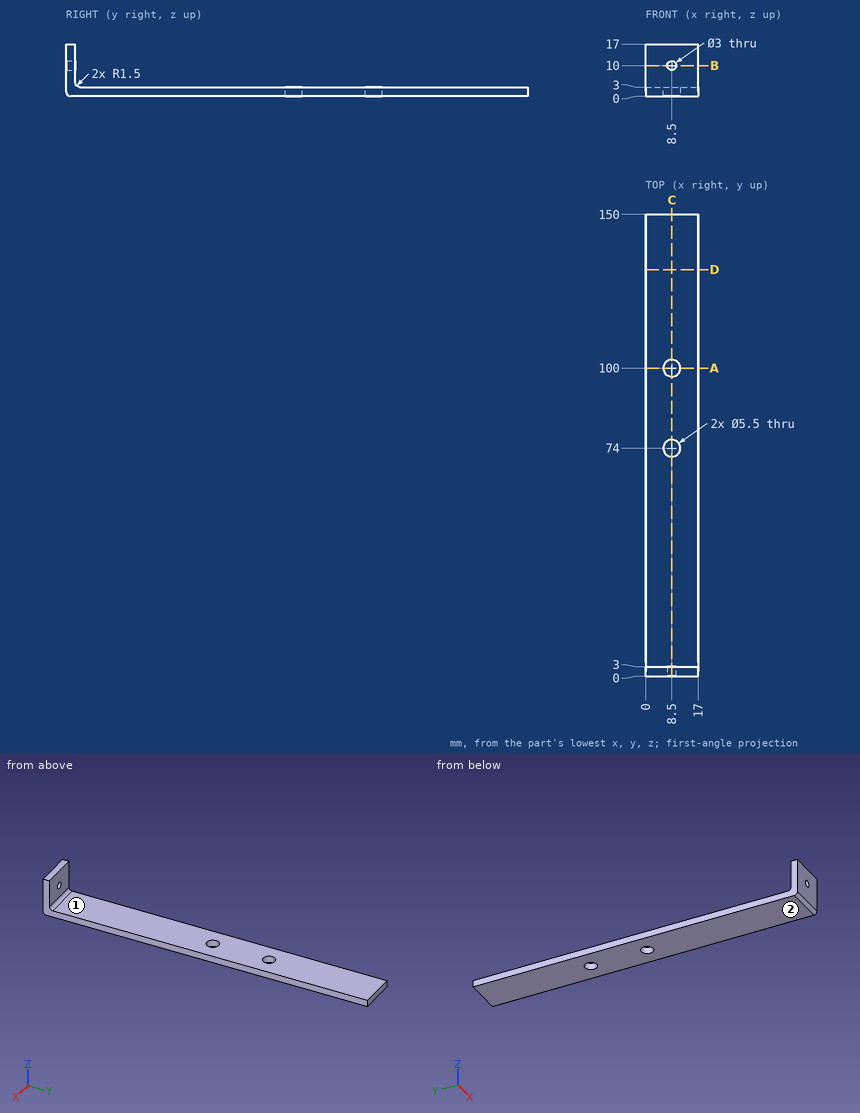
Design review of the part shown in the three views and the two pictorial views. Dimensions are in mm from the part's minimum x, y and z. A direction names the side the tool comes from. Coordinates: 2 decimals unless noted, no trailing zeros. Loops run counter-clockwise (first coordinate to the right, second up) from the corner with the lowest first, then second, coordinate; pieces in that order, holes last. Notation, with made-up numbers: (-15, -15.5) - (-8, -15.5) arc R24 cw to (-8, -3.5) - close; hole circle Ø10 at (10, -6.75). An arc over 180 degrees is marked (long way). Use a Markdown table: item, result. Add a question column.
Item 1: We need section C-C (x = 8.5). Give the boundary of the cut face in (y, z).
Item 2: We need section A-A (y = 100). Give the boundary of the cut face in (x, z), and give its area (3 significant figures).
Item 3: We need section B-B (z = 10). Give the boundary of the cut face in (x, y).
Item 4: Insertion check: pin 1 Ø5 at (x, y) = (8.5, 74) entering from -Z; pin 2 Ø10 at (x, y) = (2, 93.5) entering from +Z; pin 3 Ø4 at (x, z) = (10.5, 13) entering from +Y. Each pin has a flat end and moves straight along its axis. Give the tip position at first contact, or say it passes through.
Item 5: We need section D-D (y = 132). Give the boundary of the cut face in (x, z), and give its area (3 significant figures).
Item 6: Tool access review of the marked faces 1 and 2: name each direction out of +Z, -Z, +X, -X, +Y, -Y from which nothing blocks a thin tool from reaching the whole face with its end or side.
Item 7: For line 1 (Z direction, x = 8.5, y = 1.5); line 2 (Y direction, x = 8.5, z = 1.1); line 3 (Y direction, x = 11, z = 5.75), list the stretches that pass through material, from the lowest coordinate up.
Results list:
| question | item | result |
|---|---|---|
| 1 | outline | (0, 1.5) arc R1.5 ccw to (1.5, 0) - (71.25, 0) - (71.25, 3) - (4.5, 3) arc R1.5 cw to (3, 4.5) - (3, 8.5) - (0, 8.5) - close; (0, 11.5) - (3, 11.5) - (3, 17) - (0, 17) - close; (76.75, 0) - (97.25, 0) - (97.25, 3) - (76.75, 3) - close; (102.75, 0) - (150, 0) - (150, 3) - (102.75, 3) - close |
| 2 | outline | (0, 0) - (5.75, 0) - (5.75, 3) - (0, 3) - close; (11.25, 0) - (17, 0) - (17, 3) - (11.25, 3) - close |
| 2 | area | 34.5 mm^2 |
| 3 | outline | (0, 0) - (7, 0) - (7, 3) - (0, 3) - close; (10, 0) - (17, 0) - (17, 3) - (10, 3) - close |
| 4 | pin 1 | passes through |
| 4 | pin 2 | stops at z = 3 |
| 4 | pin 3 | stops at y = 3 |
| 5 | outline | (0, 0) - (17, 0) - (17, 3) - (0, 3) - close |
| 5 | area | 51.0 mm^2 |
| 6 | face 1 | +Z, +X, -X, +Y |
| 6 | face 2 | -Z, +X, -X, +Y, -Y |
| 7 | line 1 | z = 0 to 8.5, 11.5 to 17 |
| 7 | line 2 | y = 0.05 to 71.25, 76.75 to 97.25, 102.75 to 150 |
| 7 | line 3 | y = 0 to 3 |
